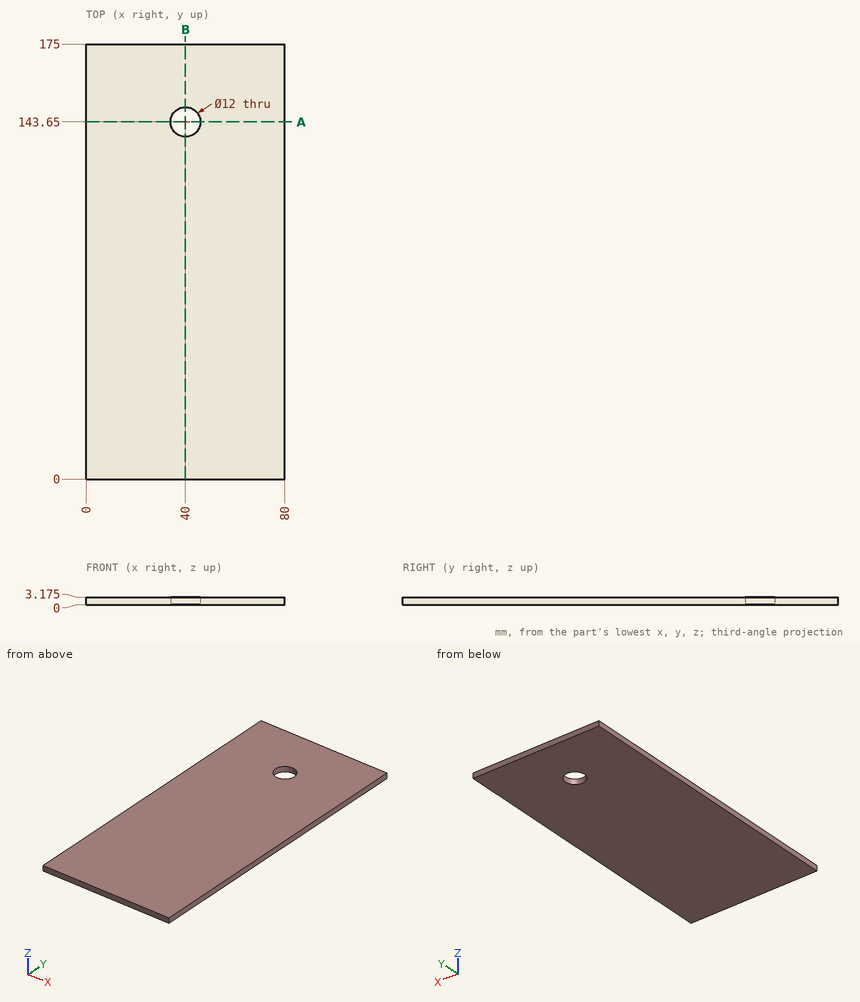
Check sheet for the drawn part. Datum: minimum x, y, z corner. Units: mm. Round coordinates to 2 decimals unless told otherwise and drop trailing zeros. Order: outer loops, then holes, each group sorted by start corner. A loop starts at its lowest first (then second) coordinate and runs counter-clockwise, first axis right, second up. Notation, with made-up numbers: (70.25, 74.5) -> (97.25, 74.5) arc R11 ccw to (97.25, 95.5) -> close; hole circle Ø3 at (68.5, 64). An arc over 180 degrees is marked (long way). Return JSON: item names as keys, results as strings. Group by question number.
Q1. Material ranges on probe 1 along Y at (x, z) = (40, 2); probe 2 along Y at (x, z) = (42, 1.1), recorded low to high. Write a range as from..to.
Q2. Section check A-A, the plane y = 143.65. Record the boundary of the cut face in (x, z) (3 decimals), plus the area to 3 significant figures.
Q3. Section check B-B, the plane x = 40. Record the boundary of the cut face in (y, z) (3 decimals).
Numbers:
{
 "1": {"probe 1": "0..137.65, 149.65..175", "probe 2": "0..137.99, 149.31..175"},
 "2": {"outline": "(0, 0) -> (34, 0) -> (34, 3.175) -> (0, 3.175) -> close; (46, 0) -> (80, 0) -> (80, 3.175) -> (46, 3.175) -> close", "area": "216 mm^2"},
 "3": {"outline": "(0, 0) -> (137.65, 0) -> (137.65, 3.175) -> (0, 3.175) -> close; (149.65, 0) -> (175, 0) -> (175, 3.175) -> (149.65, 3.175) -> close"}
}
